Geometry: final body of the model. Coordinates: model frame, mm. Give positions to 0.01 mm unless a question says otherwise; leave off trailing zeros. Write each loop counter-clockwise with the first axis right and the second up, starting at its lowest first coordinate (ties: lowest second). Pieces come first, ordered by that corner, then holes. Notation, with made-up numbers: (38.25, -26.5) - (45.25, -26.5) arc R8 ccw to (45.25, -15.5) - close; hole circle Ø10 at (6, 39). An arc over 180 degrees is marked (long way). Return JSON: item names as keys, results as strings.
from build123d import *

# Parameters (mm, degrees)
SKETCH_1_W          = 42
SKETCH_1_H          = 42
SKETCH_1_R          = 1.6
SKETCH_1_R_2        = 11
EXTRUDE_1_DEPTH     = 3
SKETCH_2_R          = 15
CUT_EXTRUDE_1_DEPTH = 30.849623113
FILLET_1_R          = 5


with BuildPart() as part:
    # 草图1 → 凸台-拉伸1 (new body)
    with BuildSketch(Plane(origin=(0, 0, 0), x_dir=(1, 0, 0), z_dir=(0, 1, 0))):
        Rectangle(SKETCH_1_W, SKETCH_1_H)
        with Locations(Location((-15.5, 15.5, 0), (0, 0, 270))):
            Circle(SKETCH_1_R, mode=Mode.SUBTRACT)
        with Locations(Location((15.5, 15.5, 0), (0, 0, 270))):
            Circle(SKETCH_1_R, mode=Mode.SUBTRACT)
        with Locations(Location((15.5, -15.5, 0), (0, 0, 270))):
            Circle(SKETCH_1_R, mode=Mode.SUBTRACT)
        with Locations(Location((-15.5, -15.5, 0), (0, 0, 270))):
            Circle(SKETCH_1_R, mode=Mode.SUBTRACT)
        with Locations(Location((0.145011043, -0.145011043, 0), (0, 0, 270))):
            Circle(SKETCH_1_R_2, mode=Mode.SUBTRACT)
    extrude(amount=EXTRUDE_1_DEPTH)

    # 草图2 → 切除-拉伸1 (cut, through all)
    with BuildSketch(Plane(origin=(0, 3, 0), x_dir=(1, 0, 0), z_dir=(0, 1, 0))):
        with Locations(Location((0, 0, 0), (0, 0, 270))):
            Circle(SKETCH_2_R)
    extrude(amount=-CUT_EXTRUDE_1_DEPTH, mode=Mode.SUBTRACT)

    # 圆角1
    fillet_1_edges = [part.edges().sort_by_distance(p)[0] for p in [
        (-21, 1.5, 21),
        (-21, 1.5, -21),
        (21, 1.5, -21),
        (21, 1.5, 21),
    ]]
    fillet(fillet_1_edges, radius=FILLET_1_R)


solid = part.part
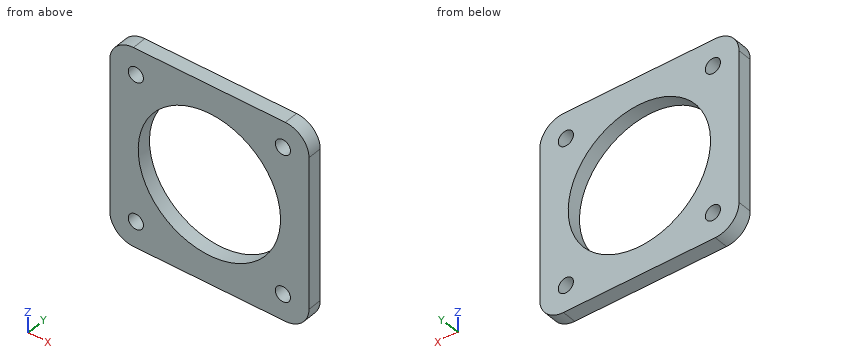
Q1. Material intervals for probe 1 along X at (y, z) = (0.75, 0); probe 2 along X at (y, z) = (1.35, 15.5); probe 3 along X at (y, z) = (2.1, 16), sorted ascending. Write a range as [from, to].
Answer key:
{"probe 1": "x = [-21, -15], [15, 21]", "probe 2": "x = [-21, -17.1], [-13.9, 13.9], [17.1, 21]", "probe 3": "x = [-21, -17.02], [-13.98, 13.98], [17.02, 21]"}
Q2. Section query B-B, the plane z = 15.5. Return the cut outline in (x, y).
Answer key:
{"outline": "(-21, 0) - (-17.1, 0) - (-17.1, 3) - (-21, 3) - close; (-13.9, 0) - (13.9, 0) - (13.9, 3) - (-13.9, 3) - close; (17.1, 0) - (21, 0) - (21, 3) - (17.1, 3) - close"}
Q3. Section query A-A, the plane x = 0. Return the cut outline in (y, z).
Answer key:
{"outline": "(0, -21) - (3, -21) - (3, -15) - (0, -15) - close; (0, 15) - (3, 15) - (3, 21) - (0, 21) - close"}
Q4. Pin query (flat end, axial travel): P1, Ø4, axis at x = -15.5, z = 11, coming from the -Y side. Return the tip coordinate at first contact, or that it passes through.
Answer key:
{"P1": "stops at y = 0"}
Q5. Section query D-D, the plane y = 1.4. Return the cut outline in (x, z).
Answer key:
{"outline": "(-21, -16) arc R5 ccw to (-16, -21) - (16, -21) arc R5 ccw to (21, -16) - (21, 16) arc R5 ccw to (16, 21) - (-16, 21) arc R5 ccw to (-21, 16) - close; hole circle Ø3.2 at (-15.5, -15.5); hole circle Ø3.2 at (-15.5, 15.5); hole circle Ø30 at (0, 0); hole circle Ø3.2 at (15.5, -15.5); hole circle Ø3.2 at (15.5, 15.5)"}
Q6. Section query C-C, the plane z = 0. Return the cut outline in (x, y).
Answer key:
{"outline": "(-21, 0) - (-15, 0) - (-15, 3) - (-21, 3) - close; (15, 0) - (21, 0) - (21, 3) - (15, 3) - close"}
